Check sheet for the modelled part. Datum: model origin and axes. Units: mm. A direction names the side the tool comes from. Round coordinates to 2 decimals unless told otherwise and drop trailing zeros. Write each loop counter-clockwise with the first axis right and the second up, starting at its lowest first coordinate (ties: lowest second). Pieces come first, ordered by that corner, then holes. Notation, with made-up numbers: (42, 19) -> (51, 19) arc R24 ccw to (51, 31) -> close; hole circle Ø11 at (-11, 33.5). An arc over 180 degrees is marked (long way). Write item = value, one per line.
from build123d import *

# Parameters (mm, degrees)
F1_DEPTH = 2
F0_R     = 3
F0_R_2   = 1.5
F2_DEPTH = 5
F4_DEPTH = 5
F5_DEPTH = 8
F6_DEPTH = 4
F7_DEPTH = 15


with BuildPart() as f1:
    # F0 (on Top) → F1 (new body)
    with BuildSketch(Plane.XY):
        with BuildLine():
            Line((-14, -20), (-2.69212803, -20))
            ThreePointArc((-2.69212803, -20), (0, -18.323800087), (2.69212803, -20))
            Line((2.69212803, -20), (14, -20))
            ThreePointArc((14, -20), (14.7071067812, -19.7071067812), (15, -19))
            Line((15, -19), (15, -15.5))
            ThreePointArc((15, -15.5), (14.4142135624, -16.9142135624), (13, -17.5))
            Line((13, -17.5), (-13, -17.5))
            ThreePointArc((-13, -17.5), (-14.4142135624, -16.9142135624), (-15, -15.5))
            Line((-15, -15.5), (-15, -19))
            ThreePointArc((-15, -19), (-14.7071067812, -19.7071067812), (-14, -20))
        make_face()
    extrude(amount=F1_DEPTH)

    # F0 (on Top) → F2 (join)
    with BuildSketch(Plane.XY):
        with BuildLine():
            Line((2.7598104581, -22.5), (16.5, -22.5))
            ThreePointArc((16.5, -22.5), (17.9142135624, -21.9142135624), (18.5, -20.5))
            Line((18.5, -20.5), (18.5, 3.5))
            ThreePointArc((18.5, 3.5), (18.2071067812, 4.2071067812), (17.5, 4.5))
            ThreePointArc((17.5, 4.5), (16.7928932188, 4.7928932188), (16.5, 5.5))
            Line((16.5, 5.5), (16.5, 17.5694916397))
            Line((16.5, 17.5694916397), (16.5, 20.5))
            ThreePointArc((16.5, 20.5), (15.9142135624, 21.9142135624), (14.5, 22.5))
            Line((14.5, 22.5), (-16.5, 22.5))
            ThreePointArc((-16.5, 22.5), (-17.9142135624, 21.9142135624), (-18.5, 20.5))
            Line((-18.5, 20.5), (-18.5, 17.5694916397))
            Line((-18.5, 17.5694916397), (-18.5, -20.5))
            ThreePointArc((-18.5, -20.5), (-17.9142135624, -21.9142135624), (-16.5, -22.5))
            Line((-16.5, -22.5), (-2.7598104581, -22.5))
            ThreePointArc((-2.7598104581, -22.5), (-2.9989011853, -21.2426109214), (-2.69212803, -20))
            Line((-2.69212803, -20), (-14, -20))
            ThreePointArc((-14, -20), (-14.7071067812, -19.7071067812), (-15, -19))
            Line((-15, -19), (-15, -15.5))
            Line((-15, -15.5), (-15, 2.5))
            ThreePointArc((-15, 2.5), (-14.4142135624, 3.9142135624), (-13, 4.5))
            Line((-13, 4.5), (-12, 4.5))
            ThreePointArc((-12, 4.5), (-10.5857864376, 5.0857864376), (-10, 6.5))
            Line((-10, 6.5), (-10, 8.1054256072))
            ThreePointArc((-10, 8.1054256072), (-9.6405519552, 9.2493614806), (-8.6914107177, 9.9821118409))
            Line((-8.6914107177, 9.9821118409), (6.3085892823, 15.5084276303))
            ThreePointArc((6.3085892823, 15.5084276303), (8.1439358734, 15.2722933519), (9, 13.6317413967))
            Line((9, 13.6317413967), (9, 2.5))
            ThreePointArc((9, 2.5), (9.2928932188, 1.7928932188), (10, 1.5))
            Line((10, 1.5), (14, 1.5))
            ThreePointArc((14, 1.5), (14.7071067812, 1.2071067812), (15, 0.5))
            Line((15, 0.5), (15, -15.5))
            Line((15, -15.5), (15, -19))
            ThreePointArc((15, -19), (14.7071067812, -19.7071067812), (14, -20))
            Line((14, -20), (2.69212803, -20))
            ThreePointArc((2.69212803, -20), (2.9220184881, -20.6442355536), (3, -21.323800087))
            ThreePointArc((3, -21.323800087), (2.9393393283, -21.9240369676), (2.7598104581, -22.5))
        make_face()
        with BuildLine():
            ThreePointArc((-12.5, 17.5694916397), (-15.5, 14.5694916397), (-18.5, 17.5694916397))
            ThreePointArc((-18.5, 17.5694916397), (-15.5, 20.5694916397), (-12.5, 17.5694916397))
        make_face(mode=Mode.SUBTRACT)
        with Locations((13.5, 17.5694916397)):
            Circle(F0_R, mode=Mode.SUBTRACT)
        with BuildLine():
            ThreePointArc((2.69212803, -20), (0, -18.323800087), (-2.69212803, -20))
            Line((-2.69212803, -20), (-0.7053746024, -20))
            ThreePointArc((-0.7053746024, -20), (0, -19.823800087), (0.7053746024, -20))
            Line((0.7053746024, -20), (2.69212803, -20))
        make_face()
        with BuildLine():
            ThreePointArc((-2.69212803, -20), (-2.9989011853, -21.2426109214), (-2.7598104581, -22.5))
            Line((-2.7598104581, -22.5), (-0.9308886961, -22.5))
            ThreePointArc((-0.9308886961, -22.5), (-1.4939342005, -21.1890388), (-0.7053746024, -20))
            Line((-0.7053746024, -20), (-2.69212803, -20))
        make_face()
        with BuildLine():
            Line((0.9308886961, -22.5), (2.7598104581, -22.5))
            ThreePointArc((2.7598104581, -22.5), (2.9393393283, -21.9240369676), (3, -21.323800087))
            ThreePointArc((3, -21.323800087), (2.9220184881, -20.6442355536), (2.69212803, -20))
            Line((2.69212803, -20), (0.7053746024, -20))
            ThreePointArc((0.7053746024, -20), (1.2860913466, -20.5518097708), (1.5, -21.323800087))
            ThreePointArc((1.5, -21.323800087), (1.3502468375, -21.9771250275), (0.9308886961, -22.5))
        make_face()
        with BuildLine():
            ThreePointArc((-2.7598104581, -22.5), (0, -24.323800087), (2.7598104581, -22.5))
            Line((2.7598104581, -22.5), (0.9308886961, -22.5))
            ThreePointArc((0.9308886961, -22.5), (0, -22.823800087), (-0.9308886961, -22.5))
            Line((-0.9308886961, -22.5), (-2.7598104581, -22.5))
        make_face()
        with BuildLine():
            ThreePointArc((-12.5, 17.5694916397), (-15.5, 20.5694916397), (-18.5, 17.5694916397))
            ThreePointArc((-18.5, 17.5694916397), (-15.5, 14.5694916397), (-12.5, 17.5694916397))
        make_face()
        with Locations((-15.5, 17.5694916397)):
            Circle(F0_R_2, mode=Mode.SUBTRACT)
        with Locations((13.5, 17.5694916397)):
            Circle(F0_R)
        with Locations((13.5, 17.5694916397)):
            Circle(F0_R_2, mode=Mode.SUBTRACT)
    extrude(amount=F2_DEPTH)

    # F3 (on face) → F4 (join)
    with BuildSketch(Plane.XY.offset(5)):
        with BuildLine():
            ThreePointArc((-18.5, -14.5), (-18.2071067812, -15.2071067812), (-17.5, -15.5))
            Line((-17.5, -15.5), (-16, -15.5))
            ThreePointArc((-16, -15.5), (-15.2928932188, -15.2071067812), (-15, -14.5))
            Line((-15, -14.5), (-15, 2.5))
            ThreePointArc((-15, 2.5), (-14.4142135624, 3.9142135624), (-13, 4.5))
            Line((-13, 4.5), (-12, 4.5))
            ThreePointArc((-12, 4.5), (-10.5857864376, 5.0857864376), (-10, 6.5))
            Line((-10, 6.5), (-10, 8.1054256072))
            ThreePointArc((-10, 8.1054256072), (-9.6405519552, 9.2493614806), (-8.6914107177, 9.9821118409))
            Line((-8.6914107177, 9.9821118409), (-11.5, 8.9473684211))
            Line((-11.5, 8.9473684211), (-11.5, 8.5))
            ThreePointArc((-11.5, 8.5), (-11.7928932188, 7.7928932188), (-12.5, 7.5))
            Line((-12.5, 7.5), (-16.5, 7.5))
            ThreePointArc((-16.5, 7.5), (-17.9142135624, 6.9142135624), (-18.5, 5.5))
            Line((-18.5, 5.5), (-18.5, -14.5))
        make_face()
    extrude(amount=F4_DEPTH)

    # F3 (on face) → F5 (join)
    with BuildSketch(Plane.XY.offset(5)):
        with BuildLine():
            Line((4.5, 22.5), (-9.5, 22.5))
            ThreePointArc((-9.5, 22.5), (-10.9142135624, 21.9142135624), (-11.5, 20.5))
            Line((-11.5, 20.5), (-11.5, 8.9473684211))
            Line((-11.5, 8.9473684211), (-8.6914107177, 9.9821118409))
            Line((-8.6914107177, 9.9821118409), (6.3085892823, 15.5084276303))
            Line((6.3085892823, 15.5084276303), (6.5, 15.5789473684))
            Line((6.5, 15.5789473684), (6.5, 20.5))
            ThreePointArc((6.5, 20.5), (5.9142135624, 21.9142135624), (4.5, 22.5))
        make_face()
    extrude(amount=F5_DEPTH)

    # F3 (on face) → F6 (join)
    with BuildSketch(Plane.XY.offset(5)):
        with BuildLine():
            ThreePointArc((10, -19.5), (9.5, -19.6339745962), (9.1339745962, -20))
            Line((9.1339745962, -20), (14, -20))
            ThreePointArc((14, -20), (14.5, -19.8660254038), (14.8660254038, -19.5))
            Line((14.8660254038, -19.5), (10, -19.5))
        make_face()
        with BuildLine():
            ThreePointArc((9, -21.5), (9.2928932188, -22.2071067812), (10, -22.5))
            Line((10, -22.5), (16.5, -22.5))
            ThreePointArc((16.5, -22.5), (17.9142135624, -21.9142135624), (18.5, -20.5))
            ThreePointArc((18.5, -20.5), (18.2071067812, -19.7928932188), (17.5, -19.5))
            Line((17.5, -19.5), (14.8660254038, -19.5))
            ThreePointArc((14.8660254038, -19.5), (14.5, -19.8660254038), (14, -20))
            Line((14, -20), (9.1339745962, -20))
            ThreePointArc((9.1339745962, -20), (9.0340741737, -20.2411809549), (9, -20.5))
            Line((9, -20.5), (9, -21.5))
        make_face()
    extrude(amount=-F6_DEPTH)

    # F3 (on face) → F7 (join)
    with BuildSketch(Plane.XY.offset(5)):
        with BuildLine():
            ThreePointArc((10, -19.5), (9.5, -19.6339745962), (9.1339745962, -20))
            Line((9.1339745962, -20), (14, -20))
            ThreePointArc((14, -20), (14.5, -19.8660254038), (14.8660254038, -19.5))
            Line((14.8660254038, -19.5), (10, -19.5))
        make_face()
        with BuildLine():
            ThreePointArc((9, -21.5), (9.2928932188, -22.2071067812), (10, -22.5))
            Line((10, -22.5), (16.5, -22.5))
            ThreePointArc((16.5, -22.5), (17.9142135624, -21.9142135624), (18.5, -20.5))
            ThreePointArc((18.5, -20.5), (18.2071067812, -19.7928932188), (17.5, -19.5))
            Line((17.5, -19.5), (14.8660254038, -19.5))
            ThreePointArc((14.8660254038, -19.5), (14.5, -19.8660254038), (14, -20))
            Line((14, -20), (9.1339745962, -20))
            ThreePointArc((9.1339745962, -20), (9.0340741737, -20.2411809549), (9, -20.5))
            Line((9, -20.5), (9, -21.5))
        make_face()
    extrude(amount=F7_DEPTH)


solid = f1.part
(1) Material ranges on L1, parallel to Y at x = 13.5, z = 2.1; L2, parallel to X at y = 0, z = 2; L3, parallel to Y at x = 13.5, z = 1.35, recorded low to high. Write a range as [from, to].
Worked answers:
L1 = [-22.5, -19.5], [1.5, 16.07], [19.07, 22.5]
L2 = [-18.5, -15], [15, 18.5]
L3 = [-22.5, -17.44], [1.5, 16.07], [19.07, 22.5]
(2) Sectioned sample at C-C on x = -4.5. Enter the section's corners in (y, z), then the cut area to 3 significant figures.
Worked answers:
outline = (-22.5, 0) -> (-17.5, 0) -> (-17.5, 2) -> (-20, 2) -> (-20, 5) -> (-22.5, 5) -> close; (11.53, 0) -> (22.5, 0) -> (22.5, 13) -> (11.53, 13) -> close
area = 160 mm²
(3) Release check for a two-part mould opening along X. For faces 1 (the flat face through (-12.5, 4.5, 4.9)), 2 (the cylindrical face through (0.047, -18.324, 3.479)), 3 (the flat face through (16.5, 13, 2)), 4 (the flat face through (-16, -3, 10)) record: pulls with the +X half, pulls with the -X half, needs draft (parallel to the pull), parting line crosses it, or undercut.
Worked answers:
face_1 = undercut
face_2 = undercut
face_3 = pulls with the +X half
face_4 = needs draft
(4) Access from +Z, -Z, +X, -X, +Y, -Y to the whole of each face (thin tool, end or side, straight path). Record for faces 5 (the flat face through (-11.5, 15, 9)), 6 (the flat face through (9, -21, 12)), 7 (the cylindrical face through (-18.215, -15.199, 7.465)).
Worked answers:
face_5 = +Z, -X, +Y
face_6 = +Z, -X, +Y, -Y
face_7 = +Z, -X, -Y
(5) Sectioned sample at A-A on z = 6.25. Enter the section's corners in (x, y).
Worked answers:
outline = (-18.5, -14.5) arc R1 ccw to (-17.5, -15.5) -> (-16, -15.5) arc R1 ccw to (-15, -14.5) -> (-15, 2.5) arc R2 cw to (-13, 4.5) -> (-12, 4.5) arc R2 ccw to (-10, 6.5) -> (-10, 8.11) arc R2 cw to (-8.69, 9.98) -> (6.5, 15.58) -> (6.5, 20.5) arc R2 ccw to (4.5, 22.5) -> (-9.5, 22.5) arc R2 ccw to (-11.5, 20.5) -> (-11.5, 8.5) arc R1 cw to (-12.5, 7.5) -> (-16.5, 7.5) arc R2 ccw to (-18.5, 5.5) -> close; (9, -21.5) arc R1 ccw to (10, -22.5) -> (16.5, -22.5) arc R2 ccw to (18.5, -20.5) arc R1 ccw to (17.5, -19.5) -> (10, -19.5) arc R1 ccw to (9, -20.5) -> close
(6) Sectioned sample at B-B on y = 12. Enter the section's corners in (x, z), then the cut area to 3 significant figures.
Worked answers:
outline = (-18.5, 0) -> (-3.21, 0) -> (-3.21, 13) -> (-11.5, 13) -> (-11.5, 5) -> (-18.5, 5) -> close; (9, 0) -> (16.5, 0) -> (16.5, 5) -> (9, 5) -> close
area = 180 mm²
(7) Go/stop test with flat-tipped pins: P1, Ø6.5, axis at y = 15, z = 10, coming from the -X side; P2, Ø2.5, axis at y = 18, z = 11, coming from the +X side; P3, Ø1.1, axis at x = -12.5, z = 6, coming from the -Y side. Record where each tip stops, or that it passes through.
Worked answers:
P1 = -11.5
P2 = 6.5
P3 = 4.5
